Autodesk Inventor part; units mm, degrees
ref_plane "YZ Plane" through (0, 0, 0) normal (1, 0, 0) x (0, 1, 0)
ref_plane "XZ Plane" through (0, 0, 0) normal (0, 1, 0) x (-1, 0, 0)
ref_plane "XY Plane" through (0, 0, 0) normal (0, 0, 1) x (1, 0, 0)
sketch "Skizze1" plane through (0, 0, 0) normal (0, 1, 0) x (-1, 0, 0)
  line L0 (9.105, 12) -> (-9.105, 12)
  line L1 (-9.105, 12) -> (-9.105, -12)
  line L2 (-9.105, -12) -> (9.105, -12)
  line L3 (9.105, -12) -> (9.105, 12)
  line L4 (9.105, 12) -> (-9.105, -12) construction
  line L5 (-9.105, 12) -> (9.105, -12) construction
  point P0 (0, 0)
  dimension "d0" = 18.21
  dimension "d1" = 24
extrude "Extrusion1" add sketch "Skizze1" along normal blind 3.5
sketch "Skizze2" plane through (0, 3.5, 0) normal (0, 1, 0) x (1, 0, 0)
  line L0 (9.105, -12) -> (9.105, 12)
  line L1 (9.105, 12) -> (-9.105, 12)
  line L2 (9.105, -12) -> (5.195, -12)
  line L3 (5.195, -12) -> (5.195, 12)
  line L4 (5.195, 12) -> (9.105, 12)
  line L5 (9.105, 12) -> (9.105, -12)
  line L6 (9.105, -12) -> (9.105, 12)
  line L7 (9.105, 12) -> (-9.105, 12)
  line L8 (-9.105, 12) -> (-9.105, -12)
  line L9 (-9.105, -12) -> (9.105, -12)
  point P0 (0, 0)
  dimension "d4" = 3.91
extrude "Extrusion2" cut sketch "Skizze2" against normal through all contours L9 L8 L1 L3
sketch "Skizze3" plane through (0, 3.5, 0) normal (0, 1, 0) x (1, 0, 0)
  line L0 (13.39, -9.55) -> (-3, -9.55)
  line L1 (-3, -9.55) -> (-3, 9.55)
  line L2 (-3, 9.55) -> (13.39, 9.55)
  line L3 (13.39, 9.55) -> (13.39, -9.55)
  line L4 (5.195, 12) -> (5.195, -12)
  line L5 (13.39, -9.55) -> (-3, 9.55) construction
  line L6 (-3, -9.55) -> (13.39, 9.55) construction
  line L7 (9.105, -12) -> (9.105, 12)
  line L8 (9.105, -9.55) -> (-9.105, -9.55)
  line L9 (-9.105, -9.55) -> (-9.105, -12.55)
  line L10 (-9.105, -12.55) -> (9.105, -12.55)
  line L11 (9.105, -12.55) -> (9.105, -9.55)
  line L12 (9.105, 9.55) -> (-9.105, 9.55)
  line L13 (-9.105, 9.55) -> (-9.105, 12.55)
  line L14 (-9.105, 12.55) -> (9.105, 12.55)
  line L15 (9.105, 12.55) -> (9.105, 9.55)
  point P0 (0, 0)
  point P1 (5.195, 0)
  dimension "d7" = 19.1
  dimension "d8" = 18.21
  dimension "d9" = 3
  dimension "d10" = 18.21
  dimension "d11" = 3
extrude "Extrusion3" add sketch "Skizze3" along normal blind 3 contours L7 L11 L10 L9 L8 L0 | L2 L12 L13 L14 L15 L7
sketch "Skizze4" plane through (0, 3.5, 0) normal (0, -1, 0) x (1, 0, 0)
  line L0 (5.195, 12) -> (9.105, 12)
  line L1 (9.105, 12.55) -> (9.105, 12)
  line L2 (-9.105, 12.55) -> (9.105, 12.55)
  line L3 (-9.105, 9.55) -> (-9.105, 12.55)
  line L4 (5.195, 9.55) -> (-9.105, 9.55)
  line L5 (5.195, 9.55) -> (5.195, 12)
  line L6 (5.195, -12) -> (5.195, -9.55)
  line L7 (-9.105, -9.55) -> (5.195, -9.55)
  line L8 (-9.105, -12.55) -> (-9.105, -9.55)
  line L9 (9.105, -12.55) -> (-9.105, -12.55)
  line L10 (9.105, -12) -> (9.105, -12.55)
  line L11 (9.105, -12) -> (5.195, -12)
  line L12 (9.105, 12.55) -> (9.105, 12)
  line L13 (9.105, 12.55) -> (5.195, 12.55)
  line L14 (5.195, 12.55) -> (5.195, 9.55)
  line L15 (5.195, 9.55) -> (9.105, 9.55)
  line L16 (9.105, 9.55) -> (9.105, 12.55)
  line L17 (9.105, -12.55) -> (-9.105, -12.55)
  line L18 (5.195, -9.55) -> (5.195, 9.55)
  line L19 (9.105, -12.55) -> (5.195, -12.55)
  line L20 (5.195, -12.55) -> (5.195, -9.55)
  line L21 (5.195, -9.55) -> (9.105, -9.55)
  line L22 (9.105, -9.55) -> (9.105, -12.55)
  point P0 (0, 0)
extrude "Extrusion4" add sketch "Skizze4" along normal up to surface (3.5 mm away) contours L14 L2 L1 L0 | L0 L16 L15 L5 | L21 L22 L11 L6 | L11 L10 L9 L20
sketch "Skizze5" plane through (9.105, 0, 12.55) normal (1, 0, 0) x (0, 0, -1)
  line L0 (0, 3.5) -> (0, 0)
  line L1 (0, 0) -> (25.1, 0)
  line L2 (25.1, 0) -> (25.1, 6.5)
  line L3 (25.1, 6.5) -> (0, 6.5)
  line L4 (0, 6.5) -> (0, 0)
  point P0 (12.55, 0)
extrude "Extrusion5" add sketch "Skizze5" along normal blind 2
properties part number "CentrationTool"
The model under review builds one solid part; all positions refer to its coordinate system, in mm. A direction names the side the tool comes from. Give positions to 0.01 mm unless a question says otherwise; leave off trailing zeros. Loops run counter-clockwise (first coordinate to the right, second up) from the corner with the lowest first, then second, coordinate; pieces in that order, holes last. Notation, with made-up numbers: (13.25, -33) -> (31.25, -33) arc R20 ccw to (31.25, -12) -> close; hole circle Ø8 at (67, -36). An arc over 180 degrees is marked (long way). Answer as a JSON object with one key per item and string values. Group by question number.
Q1. Wall thickness on line 1 along Z through (x, y) = (-1.5, 6); line 2 along X through (y, z) = (1.5, -8) (3 decimals); line 3 along X through (y, z) = (5.5, 3.75) (3 decimals): over which ranges is each line inside the solid? List them lowest first.
Q2. Take a section at C-C (x = 5.5). Write out the cut boundary in (y, z), plus the area to 3 significant figures.
Q3. Tool access review of faces 1 (the flat face through (-2, 3.5, 11)), 2 (the flat face through (0, 5, 9.55)), 3 (the flat face through (-9.105, 5, -11)): name each direction out of +Z, -Z, +X, -X, +Y, -Y from which nothing blocks a thin tool from reaching the whole face with its end or side.
Q4. Insertion check: pin 1 (1.5 mm diameter, centred on x = -0.5, z = 11.5, fed in from -Y); pin 2 (3.5 mm diameter, centred on y = 5.5, z = 1.5, fed in from -X) (3 decimals); pin 3 (1.8 mm diameter, centred on y = 1.5, z = 1, fed in from -X) (3 decimals). Each pin has a flat end and moves straight along its axis. Give the tip position at first contact, or say it passes through.
Q5. Take a section at B-B (y = 5). Write out the cut boundary in (x, z) (3 decimals).
Q6. Draft analysis for pull direction Z (two halves, no side actions). For faces 4 (the flat face through (7, 3.5, 0)), 5 (the flat face through (3, 4, 12.55)), 6 (the flat face through (3, 4, -12.55)), 7 (the flat face through (5.195, 2, 0)), state which applies: pulls with the +Z half, pulls with the -Z half, needs draft (parallel to the pull), parting line crosses it, or undercut.
Q7. Take a section at D-D (z = 2.75). Write out the cut boundary in (x, y) (3 decimals), plus the area to 3 significant figures.
Q8. Take a section at A-A (x = -5.5). Write out the cut boundary in (y, z), plus the area to 3 significant figures.
Answer below:
{
 "1": {"line 1": "z = -12.55 to -9.55, 9.55 to 12.55", "line 2": "x = 5.195 to 11.105", "line 3": "x = 9.105 to 11.105"},
 "2": {"outline": "(0, -12.55) -> (6.5, -12.55) -> (6.5, -9.55) -> (3.5, -9.55) -> (3.5, 9.55) -> (6.5, 9.55) -> (6.5, 12.55) -> (0, 12.55) -> close", "area": "106 mm2"},
 "3": {"face 1": "+Z, -Z, -X, -Y", "face 2": "-X, +Y", "face 3": "+Z, -Z, -X, +Y, -Y"},
 "4": {"pin 1": "stops at y = 3.5", "pin 2": "stops at x = 9.105", "pin 3": "stops at x = 5.195"},
 "5": {"outline": "(-9.105, -12.55) -> (11.105, -12.55) -> (11.105, 12.55) -> (-9.105, 12.55) -> (-9.105, 9.55) -> (9.105, 9.55) -> (9.105, -9.55) -> (-9.105, -9.55) -> close"},
 "6": {"face 4": "undercut", "face 5": "pulls with the +Z half", "face 6": "pulls with the -Z half", "face 7": "needs draft"},
 "7": {"outline": "(5.195, 0) -> (11.105, 0) -> (11.105, 6.5) -> (9.105, 6.5) -> (9.105, 3.5) -> (5.195, 3.5) -> close", "area": "26.7 mm2"},
 "8": {"outline": "(3.5, -12.55) -> (6.5, -12.55) -> (6.5, -9.55) -> (3.5, -9.55) -> close; (3.5, 9.55) -> (6.5, 9.55) -> (6.5, 12.55) -> (3.5, 12.55) -> close", "area": "18.0 mm2"}
}
